Can you work these out from the model? Positions are in its coordinate system, mm. A direction names the side the tool comes from. Give positions to 0.01 mm unless a question says otherwise; leave off trailing zeros. Loops run counter-clockwise (first coordinate to the right, second up) from the corner with the lowest first, then second, coordinate; pieces in that order, holes last.
from build123d import *

# Parameters (mm, degrees)
SKETCH1_W           = 25.4
SKETCH1_H           = 63.5
BOSS_EXTRUDE1_DEPTH = 3.175
FILLET1_R           = 5.08
SKETCH2_R           = 1.5875
CUT_EXTRUDE1_DEPTH  = 3.175


with BuildPart() as part:
    # Sketch1 → Boss-Extrude1 (new body)
    with BuildSketch(Plane.XY):
        with BuildLine():
            ThreePointArc((-36.600968343, 63.5), (-69.85, 50.8), (-36.600968343, 38.1))
            Line((-36.600968343, 38.1), (-50.8, 38.1))
            Line((-50.8, 38.1), (-50.8, 63.5))
            Line((-50.8, 63.5), (-36.600968343, 63.5))
        make_face()
        with BuildLine():
            Line((-50.8, 38.1), (-36.600968343, 38.1))
            ThreePointArc((-36.600968343, 38.1), (-33.004016562, 44.00253919), (-31.75, 50.8))
            ThreePointArc((-31.75, 50.8), (-33.004016562, 57.59746081), (-36.600968343, 63.5))
            Line((-36.600968343, 63.5), (-50.8, 63.5))
            Line((-50.8, 63.5), (-50.8, 38.1))
        make_face()
        with BuildLine():
            Line((-36.600968343, 38.1), (-25.4, 38.1))
            Line((-25.4, 38.1), (-25.4, 63.5))
            Line((-25.4, 63.5), (-36.600968343, 63.5))
            ThreePointArc((-36.600968343, 63.5), (-33.004016562, 57.59746081), (-31.75, 50.8))
            ThreePointArc((-31.75, 50.8), (-33.004016562, 44.00253919), (-36.600968343, 38.1))
        make_face()
        with Locations((-12.7, 31.75)):
            Rectangle(SKETCH1_W, SKETCH1_H)
    extrude(amount=BOSS_EXTRUDE1_DEPTH)

    # Fillet1
    fillet1_edges = [part.edges().sort_by_distance(p)[0] for p in [
        (0, 63.5, 1.5875),
        (0, 0, 1.5875),
        (-25.4, 0, 1.5875),
        (-25.4, 38.1, 1.5875),
    ]]
    fillet(fillet1_edges, radius=FILLET1_R)

    # Sketch2 → Cut-Extrude1 (cut)
    with BuildSketch(Plane.XY.offset(3.175)):
        with Locations((-6.35, 50.8)):
            Circle(SKETCH2_R)
        with Locations((-12.7, 50.8)):
            Circle(SKETCH2_R)
        with Locations((-19.05, 50.8)):
            Circle(SKETCH2_R)
        with Locations((-25.4, 50.8)):
            Circle(SKETCH2_R)
        with Locations((-31.75, 50.8)):
            Circle(SKETCH2_R)
        with Locations((-38.1, 50.8)):
            Circle(SKETCH2_R)
        with Locations((-44.45, 50.8)):
            Circle(SKETCH2_R)
        with Locations((-50.8, 50.8)):
            Circle(SKETCH2_R)
        with Locations((-57.15, 50.8)):
            Circle(SKETCH2_R)
        with Locations((-63.5, 50.8)):
            Circle(SKETCH2_R)
    extrude(amount=-CUT_EXTRUDE1_DEPTH, mode=Mode.SUBTRACT)


solid = part.part
(1) Thinking about a two-plate mould opening in X: for faces 1 (the cylindrical face through (-46.036, 50.87, 1.61)), 2 (the cylindrical face through (-1.449, 61.972, 1.61)), 3 (the flat face through (-13, 0, 2)), which applies, pulls with the +X half, pulls with the -X half, needs draft (parallel to the pull), parting line crosses it, or undercut?
Returned:
face 1: undercut
face 2: pulls with the +X half
face 3: needs draft
(2) Suppose I cut it at A-A on z = 1.15. Give the number of separate pieces and of enclosed holes in the cut face, plus the area to 3 significant figures.
Returned:
separate pieces: 1
enclosed holes: 10
area: 2,860 mm2
(3) Please list where these lines run through material, in increasing order: probe 1 along Y at (x, z) = (-50.8, 2.2); probe 2 along X at (y, z) = (14.5, 1.85); probe 3 along Y at (x, z) = (-57.15, 1.6).
Returned:
probe 1: y = 31.75 to 49.21, 52.39 to 69.85
probe 2: x = -25.4 to 0
probe 3: y = 32.84 to 49.21, 52.39 to 68.76
(4) Will these pins go through, and if not, where does the flat tip stop? P1, Ø2.5, axis at x = -38.1, y = 50.8, coming from the +Z side; P2, Ø1.6, axis at x = -32, z = 1.5, coming from the -Y side; P3, Ø1.5, axis at y = 60.5, z = 1.5, coming from the +X side; P4, Ø1.6, axis at x = -19, z = 2.5, coming from the +Y side.
Returned:
P1: passes through
P2: stops at y = 38.1
P3: stops at x = -0.18
P4: stops at y = 63.5
(5) Which directions (+Z, -Z, +X, -X, +Y, -Y) give clear straight access to the entire face, cutting with the end or side of a thin tool? Please do faces 4 (the flat face through (-34, 38.1, 2)), 5 (the cylindrical face through (-69.84, 51.44, 1.57)).
Returned:
face 4: +Z, -Z, -Y
face 5: +Z, -Z
(6) Suppose I cut it at B-B on x = -63. List the corners of the cut face in (y, z) for me (3 decimals), plus the area to 3 significant figures.
Returned:
outline: (36.169, 0) - (49.293, 0) - (49.293, 3.175) - (36.169, 3.175) - close; (52.307, 0) - (65.431, 0) - (65.431, 3.175) - (52.307, 3.175) - close
area: 83.3 mm2
